Autodesk Fusion 360 part; units mm, degrees
sketch "Sketch1" plane through (0, 0, 0) normal (0, 0, 1) x (1, 0, 0)
  line L0 (-50, 0) -> (50, 0) construction
  line L1 (0, 50) -> (0, -50) construction
  arc A0 (-50, 15) -> (-15, 50) centre (-50, 50) ccw
  arc A1 (15, 50) -> (50, 15) centre (50, 50) ccw
  arc A2 (50, -15) -> (15, -50) centre (50, -50) ccw
  arc A3 (-15, -50) -> (-50, -15) centre (-50, -50) ccw
  arc A4 (-50, 15) -> (-50, -15) centre (-50, 0) ccw
  arc A5 (15, 50) -> (-15, 50) centre (0, 50) ccw
  arc A6 (50, -15) -> (50, 15) centre (50, 0) ccw
  arc A7 (-15, -50) -> (15, -50) centre (0, -50) ccw
  dimension "d2" = 100
  dimension "d3" = 100
  dimension "d4" = 30
ref_plane "WorkPlane1" through (0, 0, 30) normal (0, 0, 1) x (1, 0, 0)
sketch "Sketch2" plane through (0, 0, 30) normal (0, 0, 1) x (1, 0, 0)
  circle A0 centre (0, 0) radius 20
loft "Loft1" add profiles "Sketch1", "Sketch2" section 1 section 2
sketch "Sketch3" plane through (0, 0, 30) normal (0, 0, 1) x (-1, 0, 0)
  circle A0 centre (0, 0) radius 20
  circle A1 centre (0, 0) radius 11.05
  dimension "d6" = 22.1
extrude "Extrude1" cut sketch "Sketch3" against normal blind 7 contours A1
Model file for the job. Use its own axes, mm. Coordinates: 2 decimals unless noted, no trailing zeros. Return JSON: item names as keys, results as strings. Group by question number.
1) Probe line 1 (Y direction, x = 0, z = 24.5); line 2 (X direction, y = 0, z = 26); line 3 (Y direction, x = 0, z = 25.5). List the from-to ranges inside material, lowest first. Write a range as from..to.
2) Mould opens along X. For faces 1 (the cylindrical face through (2.395, 10.787, 26.549)), 2 (the flat face through (1, 1, 0)), 3 (the flat face through (0, 0, 23)) say: released by +X, released by -X, zero draft, split by the parting line, or undercut.
3) Flat gauge pins, fed straight in: P1, Ø1.5, axis at y = -14, z = 13, coming from the -X side; P2, Ø1, axis at y = -41.5, z = 12, coming from the -X side; P3, Ø10, axis at x = 38.5, z = 16.5, coming from the +Y side; P4, Ø2, axis at x = -6.5, y = -48.5, coming from the -Z side. Where does each tip first touch, or does it go through?
Values found:
{
 "1": {"line 1": "y = -28.25..-11.05, 11.05..28.25", "line 2": "x = -26..-11.05, 11.05..26", "line 3": "y = -26.75..-11.05, 11.05..26.75"},
 "2": {"face 1": "undercut", "face 2": "zero draft", "face 3": "undercut"},
 "3": {"P1": "stops at x = -30.7", "P2": "stops at x = -10.46", "P3": "stops at y = 11.62", "P4": "stops at z = 0"}
}
